Can you work these out from the model? Positions are in its coordinate system, mm. A direction names the side the tool comes from. Coordinates: 2 decimals unless noted, no trailing zeros. Answer as CSV lines item,"result".
from build123d import *

# Parameters (mm, degrees)
CHAMFER_SIZE = 0.5
SKETCH001_R  = 3.2
POCKET_DEPTH = 4


with BuildPart() as part:
    # Sketch → Revolution (revolve)
    with BuildSketch(Plane.XZ):
        with BuildLine():
            Line((-63.5, 0), (-9, 0))
            Line((-9, 0), (-9, 6.5))
            Line((-9, 6.5), (-8, 7.5))
            Line((-8, 7.5), (0, 7.5))
            Line((0, 7.5), (0, 9))
            Line((0, 9), (-9, 9))
            ThreePointArc((-9, 9), (-12.826834, 8.238795), (-16.071068, 6.071068))
            Line((-16.071068, 6.071068), (-16.713203, 5.428932))
            ThreePointArc((-23.784271, 2.5), (-19.957437, 3.261205), (-16.713203, 5.428932))
            Line((-23.784271, 2.5), (-63, 2.5))
            Line((-63, 2.5), (-64, 1.5))
            Line((-64, 1.5), (-64, 0.5))
            Line((-64, 0.5), (-63.5, 0))
        make_face()
    revolve(axis=Axis((0, 0, 0), (0, 0, 1)))

    # Chamfer
    chamfer_edges = [part.edges().sort_by_distance(p)[0] for p in [
        (9, 0, 0),
    ]]
    chamfer(chamfer_edges, length=CHAMFER_SIZE)

    # Sketch001 (on Face13 of Chamfer) → Pocket (cut)
    with BuildSketch(Plane(origin=(0, 0, 9), x_dir=(-1, 0, 0), z_dir=(0, 0, 1))):
        with Locations((-12.990381, 7.5)):
            Circle(SKETCH001_R)
        with Locations((12.990381, 7.5)):
            Circle(SKETCH001_R)
        with Locations((0, -15)):
            Circle(SKETCH001_R)
    extrude(amount=-POCKET_DEPTH, mode=Mode.SUBTRACT)


solid = part.part
Q1. If I drill on line 1 (Z direction, x = 52, y = -14); line 2 (X direction, y = 0, z = 1.85); line 3 (X direction, y = -7.5, z = 7.55), over which ranges is the centre line in solid material (lowest first)?
Solution:
line 1,"0 to 2.5"
line 2,"-63.65 to -9, 9 to 63.65"
line 3,"-9.79 to 9.79"
Q2. For P1, Ø5, axis at y = 15, z = 7.5, coming from the +X side; P2, Ø6, axis at x = -40, y = -30.5, coming from the +Z side; P3, Ø1.6, axis at x = -1, y = 14, coming from the +Z side; P4, Ø2, axis at x = 28, z = 4, coming from the +Y side, each with a flat end and sliding along its axis, tell me the tip position at first contact or that it passes through.
Solution:
P1,"x = 9.74"
P2,"z = 2.5"
P3,"z = 5"
P4,"through"
Q3. Which directions (+Z, -Z, +X, -X, +Y, -Y) give clear straight access to the entire face, cutting with the end or side of a thin tool? Please do faces 1 (the conical face through (14.11, 7.92, 5.96)), 2 (the cylindrical face through (1.172, -8.923, 3.542)), 3 (the cylindrical face through (-10.17, -5.99, 6.43)).
Solution:
face 1,"+Z, +X"
face 2,"-Z"
face 3,"+Z"
Q4. We'd pull the mould along Y, two halves only. Please class faces 4 (the conical face through (-13.914, 8.263, 5.96)), 5 (the flat face through (0, 0, 7.5)), 6 (the flat face through (-13, -1, 0)): pulls with the +Y half, pulls with the -Y half, needs draft (parallel to the pull), parting line crosses it, or undercut.
Solution:
face 4,"parting line crosses it"
face 5,"undercut"
face 6,"needs draft"
